Can you work these out from the drawing? Everything is in mm from the part's minimum corner. A direction names the side the tool comes from. Round coordinates to 2 decimals unless told otherwise and drop trailing zeros. Write each loop counter-clockwise with the first axis right and the second up, starting at its lowest first coordinate (ties: lowest second). Pieces come first, ordered by that corner, then holes. Notation, with made-up numbers: (18.25, 74) -> (59.25, 74) arc R17 cw to (59.25, 92) -> close; hole circle Ø10 at (58.5, 45). An arc over 180 degrees is marked (long way). Answer as CSV lines item,"result".
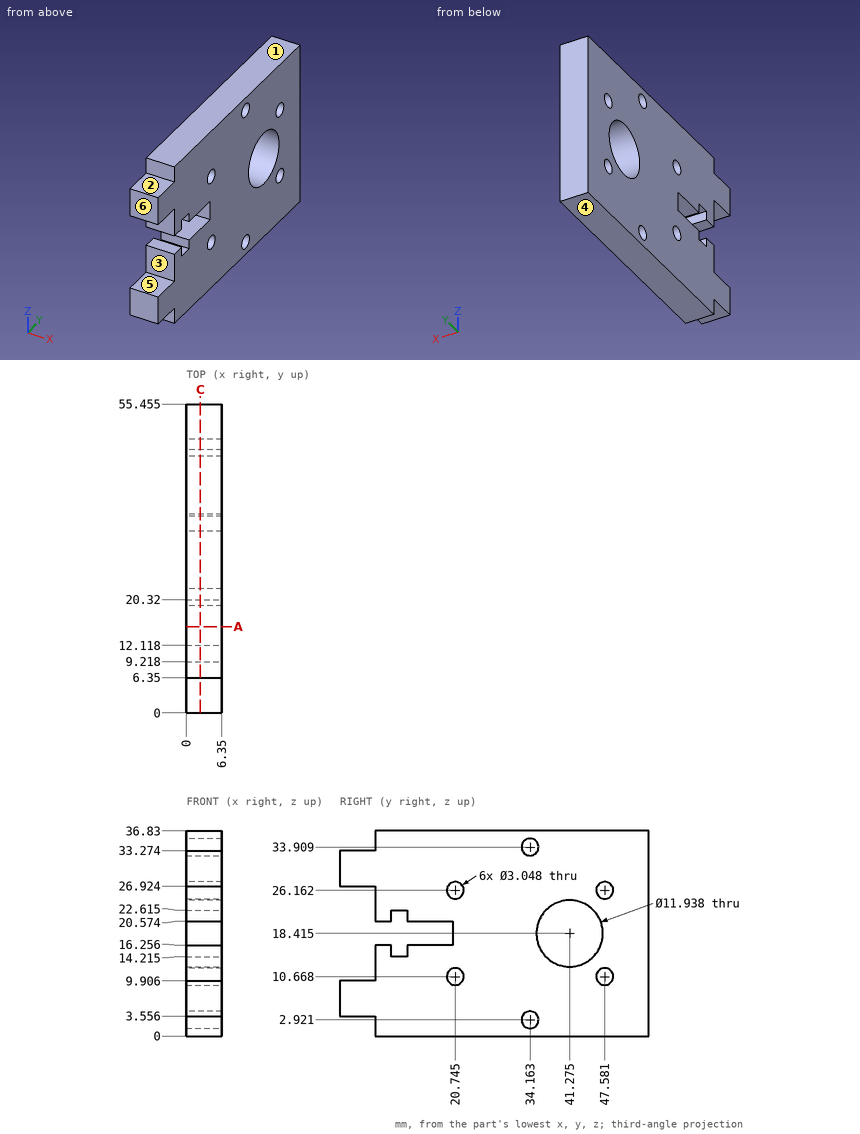
Item 1: For the marked faces 1 and 2, which set-ups out of +Z, -Z, +X, -X, +Y, -Y let a thin tool reach every point of the face, with its end or its side?
Results found:
face 1,"+Z, +X, -X, +Y, -Y"
face 2,"+Z, +X, -X, -Y"
Item 2: Suppose I cut it at C-C, the plane x = 2.5. State how many separate pieces and enclosed holes the cut face has, then the cut area to 3 significant figures.
Results found:
separate pieces,"1"
enclosed holes,"7"
area,"1,660 mm²"
Item 3: If we mould it in two halves opening along Z, with no side actions, what happens to the marked faces 3, 4, 5 and 6? For each: pulls with the +Z half, pulls with the -Z half, needs draft (parallel to the pull), parting line crosses it, or undercut.
Results found:
face 3,"undercut"
face 4,"pulls with the -Z half"
face 5,"undercut"
face 6,"needs draft"
Item 4: Will these pins go through, and if not, where does the flat tip stop? pin 1 (2 mm diameter, centred on x = 3, z = 24.5, fed in from -Y); pin 2 (3 mm diameter, centred on x = 3.5, y = 2.5, fed in from -Z).
Results found:
pin 1,"stops at y = 6.35"
pin 2,"stops at z = 3.56"
Item 5: Suppose I cut it at A-A, the plane y = 15.5. List the corners of the cut face in (x, z) for me.
Results found:
outline,"(0, 0) -> (6.35, 0) -> (6.35, 16.26) -> (0, 16.26) -> close; (0, 20.57) -> (6.35, 20.57) -> (6.35, 36.83) -> (0, 36.83) -> close"
Item 6: I need wall thicknesses on L1, parallel to Z at x = 2.75, y = 47.5; L2, parallel to Z at x = 0.5, y = 4; L3, parallel to Z at x = 5.25, y = 9. Which ranges of each line are inside material? Lowest first, please.
Results found:
L1,"z = 0 to 9.15, 12.19 to 24.64, 27.68 to 36.83"
L2,"z = 3.56 to 9.91, 26.92 to 33.27"
L3,"z = 0 to 16.26, 20.57 to 36.83"
